```python
from build123d import *

# Parameters (mm, degrees)
SKETCH1_W           = 15.8
SKETCH1_H           = 16.15
SKETCH1_W_2         = 12.2
SKETCH1_H_2         = 12.55
BOSS_EXTRUDE1_DEPTH = 3
SKETCH1_3_W         = 15.8
SKETCH1_3_H         = 16.15
BOSS_EXTRUDE2_DEPTH = 5
BOSS_EXTRUDE3_DEPTH = 6.6
BOSS_EXTRUDE4_START = 6.5
SKETCH1_5_R         = 16
SKETCH1_5_R_2       = 3.55
BOSS_EXTRUDE4_DEPTH = 6.5
SKETCH2_R           = 1.225
CUT_EXTRUDE1_DEPTH  = 12
CUT_EXTRUDE2_START  = -4.6
CUT_EXTRUDE2_DEPTH  = 4.6
CUT_EXTRUDE3_START  = -4
CUT_EXTRUDE3_DEPTH  = 4
SKETCH5_R           = 0.5
CUT_EXTRUDE4_DEPTH  = 0.4


with BuildPart() as part:
    # Sketch1 → Boss-Extrude1 (new body)
    with BuildSketch(Plane(origin=(0, 0, 0), x_dir=(1, 0, 0), z_dir=(0, 1, 0))):
        Rectangle(SKETCH1_W, SKETCH1_H)
        Rectangle(SKETCH1_W_2, SKETCH1_H_2, mode=Mode.SUBTRACT)
    extrude(amount=-BOSS_EXTRUDE1_DEPTH)

    # Sketch1<3> → Boss-Extrude2 (add)
    with BuildSketch(Plane(origin=(0, 0, 0), x_dir=(1, 0, 0), z_dir=(0, 1, 0))):
        with BuildLine():
            Line((10.7, 10.875), (-11.736028928, 10.875))
            ThreePointArc((-11.736028928, 10.875), (-15.928532305, 1.510582208), (-13.571085992, -8.475))
            Line((-13.571085992, -8.475), (10.7, -8.475))
            Line((10.7, -8.475), (10.7, 10.875))
        make_face()
        Rectangle(SKETCH1_3_W, SKETCH1_3_H, mode=Mode.SUBTRACT)
    extrude(amount=-BOSS_EXTRUDE2_DEPTH)

    # Sketch1<4> → Boss-Extrude3 (add)
    with BuildSketch(Plane(origin=(0, 0, 0), x_dir=(1, 0, 0), z_dir=(0, 1, 0))):
        with BuildLine():
            ThreePointArc((16, 0), (5.840528108, 14.895913246), (-11.736028928, 10.875))
            Line((-11.736028928, 10.875), (10.7, 10.875))
            Line((10.7, 10.875), (10.7, -8.475))
            Line((10.7, -8.475), (-13.571085992, -8.475))
            ThreePointArc((-13.571085992, -8.475), (4.408096195, -15.380789575), (16, 0))
        make_face()
    extrude(amount=-BOSS_EXTRUDE3_DEPTH)

    # Sketch1<5> → Boss-Extrude4 (add)
    with BuildSketch(Plane(origin=(0, 0, 0), x_dir=(1, 0, 0), z_dir=(0, 1, 0)).offset(BOSS_EXTRUDE4_START)):
        with Locations(Location((0, 0, 0), (0, 0, 270))):
            Circle(SKETCH1_5_R)
        with Locations(Location((0, 0, 0), (0, 0, 90))):
            Circle(SKETCH1_5_R_2, mode=Mode.SUBTRACT)
    extrude(amount=-BOSS_EXTRUDE4_DEPTH)

    # Sketch2 → Cut-Extrude1 (cut)
    with BuildSketch(Plane.XZ.offset(6.6)):
        with Locations(Location((0, 14, 0), (0, 0, 270))):
            Circle(SKETCH2_R)
        with Locations(Location((0, -14, 0), (0, 0, 270))):
            Circle(SKETCH2_R)
    extrude(amount=-CUT_EXTRUDE1_DEPTH, mode=Mode.SUBTRACT)

    # Sketch3 → Cut-Extrude2 (cut)
    with BuildSketch(Plane.XZ.offset(6.6).offset(CUT_EXTRUDE2_START)):
        with BuildLine():
            Line((-11.736028928, -10.875), (-11.736028928, 10.875))
            ThreePointArc((-11.736028928, 10.875), (-12.710331089, 9.71840952), (-13.571085992, 8.475))
            ThreePointArc((-13.571085992, 8.475), (-15.928532305, -1.510582208), (-11.736028928, -10.875))
        make_face()
    extrude(amount=CUT_EXTRUDE2_DEPTH, mode=Mode.SUBTRACT)

    # Sketch4 → Cut-Extrude3 (cut)
    with BuildSketch(Plane.XZ.offset(6.6).offset(CUT_EXTRUDE3_START)):
        with BuildLine():
            Line((10.7, 8.475), (13.571085992, 8.475))
            ThreePointArc((13.571085992, 8.475), (15.928532305, -1.510582208), (11.736028928, -10.875))
            Line((11.736028928, -10.875), (10.7, -10.875))
            Line((10.7, -10.875), (10.7, 8.475))
        make_face()
    extrude(amount=CUT_EXTRUDE3_DEPTH, mode=Mode.SUBTRACT)

    # Sketch5 → Cut-Extrude4 (cut)
    with BuildSketch(Plane.XZ.offset(2)):
        with Locations(Location((-13.736028928, 5.041127606, 0), (0, 0, 270))):
            Circle(SKETCH5_R)
        with Locations(Location((-13.736028928, 2.501127606, 0), (0, 0, 270))):
            Circle(SKETCH5_R)
        with Locations(Location((-13.736028928, -0.038872394, 0), (0, 0, 270))):
            Circle(SKETCH5_R)
        with Locations(Location((-13.736028928, -2.578872394, 0), (0, 0, 270))):
            Circle(SKETCH5_R)
        with Locations(Location((-13.736028928, -5.118872394, 0), (0, 0, 270))):
            Circle(SKETCH5_R)
    extrude(amount=-CUT_EXTRUDE4_DEPTH, mode=Mode.SUBTRACT)


solid = part.part
```
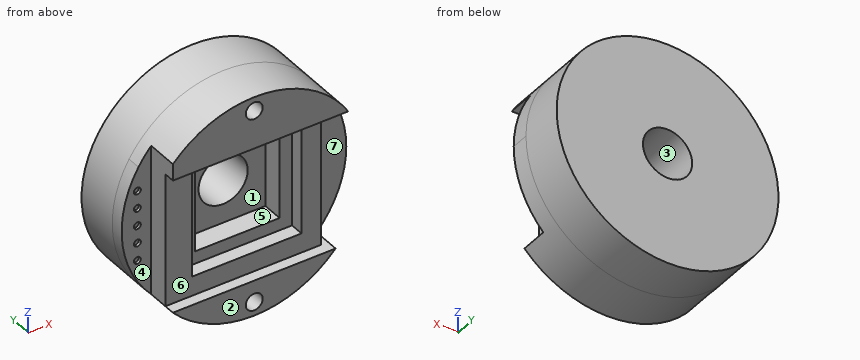
Here's how the part is built. I have some questions about the finished solid (model axes, mm). Face numbers are marked on the shaded views. A direction names the side the tool comes from. Give positions to 0.01 mm unless a question says otherwise; leave off trailing zeros. Write each loop counter-clockwise with the first axis right and the second up, starting at its lowest first coordinate (ties: lowest second). Pieces come first, ordered by that corner, then holes. Notation, with made-up numbers: (2, 14.25) -> (52, 14.25) arc R31 ccw to (52, 52.25) -> close; hole circle Ø9 at (-32.5, 77). An arc over 180 degrees is marked (long way). Write each question's results on one line, items separated by ' | '.
Item 1: On a 3-axis mill with a long thin cutter (end or side, diameter ignored), from which of +Z, -Z, +X, -X, +Y, -Y can I reach the whole of each face in a straight line? I mean the marked faces 3, 4, 5, 6 and 7. Say none if no direction works.
Output:
face 3: +Y, -Y | face 4: +Z, -Z, -X, -Y | face 5: -Y | face 6: +X, -X, -Y | face 7: +X, -Y
Item 2: If I drill on L1, parallel to Z at x = 1, y = -1.75 (3 decimals); L2, parallel to Y at x = 7.5, z = -1.5; L3, parallel to X at y = -1.5, z = 3, over which ranges is the centre line in solid material (lowest first)?
Output:
L1: z = -15.969 to -14.708, -13.292 to -6.275, 6.275 to 13.292, 14.708 to 15.969 | L2: y = -3 to 6.5 | L3: x = -15.72 to -6.1, 6.1 to 15.72
Item 3: Suppose I cut it at C-C on z = 10. Write out the boundary of the cut face in (x, y).
Output:
outline: (-12.49, -2) -> (-11.74, -2) -> (-11.74, -6.6) -> (12.49, -6.6) -> (12.49, 6.5) -> (-12.49, 6.5) -> close
Item 4: Suppose I cut it at B-B on y = 3.25. Write out the boundary of the cut face in (x, z) (3 decimals), plus the area to 3 significant figures.
Output:
outline: circle Ø32 at (0, 0); hole circle Ø7.1 at (0, 0); hole circle Ø2.45 at (0, -14); hole circle Ø2.45 at (0, 14) | area: 755 mm^2
Item 5: Suppose I cut it at D-D on x = -5.5. Write out the boundary of the cut face in (y, z) (3 decimals).
Output:
outline: (-6.6, -15.025) -> (6.5, -15.025) -> (6.5, 15.025) -> (-6.6, 15.025) -> (-6.6, 8.475) -> (-5, 8.475) -> (-5, 8.075) -> (-3, 8.075) -> (-3, 6.275) -> (0, 6.275) -> (0, -6.275) -> (-3, -6.275) -> (-3, -8.075) -> (-5, -8.075) -> (-5, -10.875) -> (-6.6, -10.875) -> close
Item 6: Suppose I cut it at A-A on x = 0. Write out the boundary of the cut face in (y, z) (3 decimals).
Output:
outline: (-6.6, -16) -> (6.5, -16) -> (6.5, -3.55) -> (0, -3.55) -> (0, -6.275) -> (-3, -6.275) -> (-3, -8.075) -> (-5, -8.075) -> (-5, -10.875) -> (-6.6, -10.875) -> (-6.6, -12.775) -> (5.4, -12.775) -> (5.4, -15.225) -> (-6.6, -15.225) -> close; (-6.6, 8.475) -> (-5, 8.475) -> (-5, 8.075) -> (-3, 8.075) -> (-3, 6.275) -> (0, 6.275) -> (0, 3.55) -> (6.5, 3.55) -> (6.5, 16) -> (-6.6, 16) -> (-6.6, 15.225) -> (5.4, 15.225) -> (5.4, 12.775) -> (-6.6, 12.775) -> close
Item 7: For pin 1 Ø1.5 at (x, y) = (6, 3.5) entering from +Z; pin 2 Ø3 at (x, y) = (8, -2) entering from +Z; pin 3 Ø1 at (x, z) = (-12, -7) entering from -Y, each with a flat end and sliding along its axis, tell me the tip position at first contact or that it passes through.
Output:
pin 1: stops at z = 15.11 | pin 2: stops at z = 14.62 | pin 3: stops at y = -5
Item 8: We'd pull the mould along Z, two halves only. Please class the marked faces 1 and 2: pulls with the +Z half, pulls with the -Z half, needs draft (parallel to the pull), parting line crosses it, or undercut.
Output:
face 1: undercut | face 2: needs draft
